Job drawing, mm, ordinate dimensions from the low corner. One solid piece. A direction names the side the tool comes from. Give positions to 0.01 mm unless a question says otherwise; leave off trailing zeros. Write each loop counter-clockwise with the first axis right and the second up, starting at its lowest first coordinate (ties: lowest second). Pieces come first, ordered by that corner, then holes. Notation, with made-up numbers: (6, 58) - (20, 58) arc R19 cw to (20, 82) - close; hole circle Ø11 at (-16, -10.75). An arc over 180 degrees is marked (long way). Use a Markdown table: item, result. Add a question column.
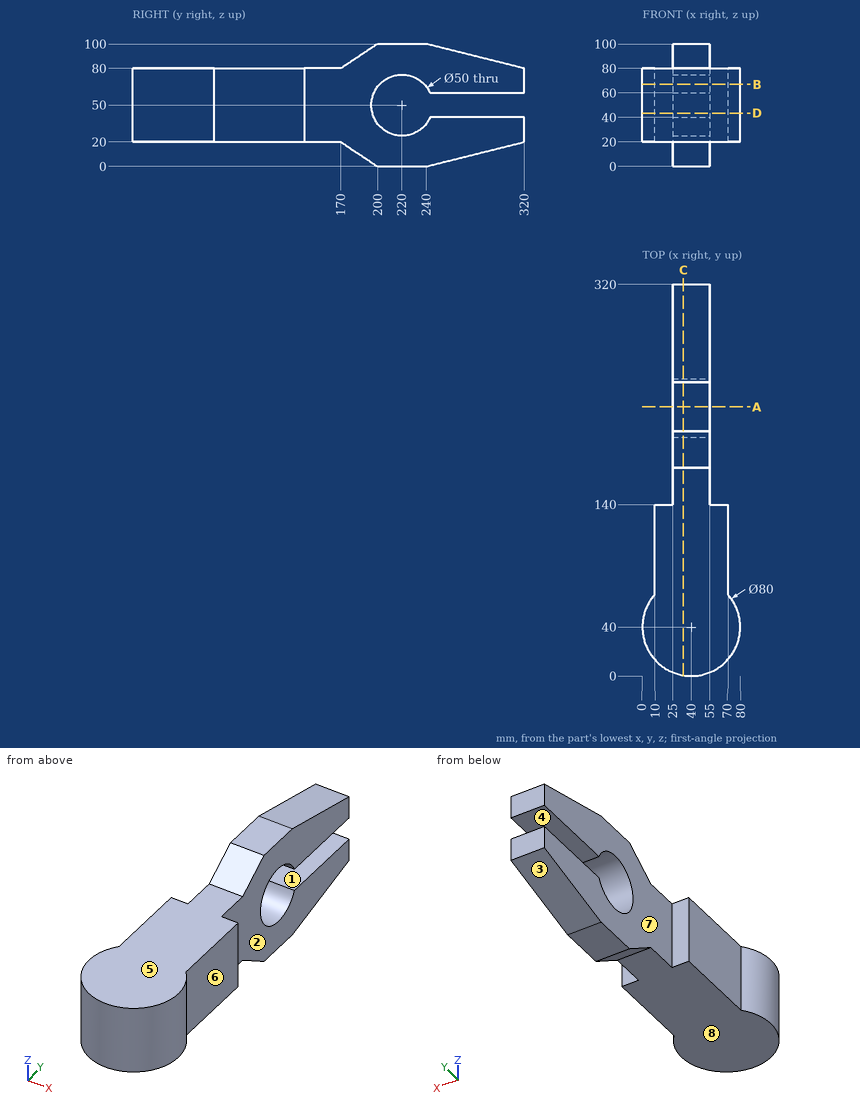
(1) Band-saw the part on A-A (y = 220). Write the cut outline in (x, z), then the cut area to 3 significant figures.
(2) Which spindle directions (+Z, -Z, +X, -X, +Y, -Y) get a long thin tool onto all of the face, cutting with end or side? Do the marked faces 4, 5, 6, 7 and 8. Say none if no direction does.
(3) Flat gauge pins, fed straight in: pin 1 (2 mm diameter, centred on y = 175, z = 23.5, fed in from -X); pin 2 (15 mm diameter, centred on x = 41, y = 293, fed in from -Z) (3 decimals); pin 3 (1.5 mm diameter, centred on x = 28.5, y = 162, fed in from +Z). Where does each tip first touch, or does it go through?
(4) Two-plate mould, pull along Z, no slides. Class the marked faces 1, 2 and 3: +Z half, -Z half, draft (parallel to the pull), parting line (faces both ways), or undercut.
(5) Probe probe 1 along Z at (x, y) = (44, 220); probe 2 along Z at (x, y) = (35.5, 165); probe 3 along X at (y, z) = (196, 62). List the from-to ranges inside material, lowest first. Write a range as [from, to].
(6) Band-saw the part on D-D (z = 43.5). Write the cut outline in (x, y), then the cut area to 3 significant figures.
(7) Band-saw the part on C-C (x = 33.5). Write the cut outline in (y, z).
(8) Band-saw the part on B-B (z = 67). Write the cut outline in (x, y).
Model answer:
| question | item | result |
|---|---|---|
| 1 | outline | (25, 0) - (55, 0) - (55, 25) - (25, 25) - close; (25, 75) - (55, 75) - (55, 100) - (25, 100) - close |
| 1 | area | 1,500 mm^2 |
| 2 | face 4 | +X, -X, +Y |
| 2 | face 5 | +Z, +X, -X, -Y |
| 2 | face 6 | +Z, -Z, +X, +Y |
| 2 | face 7 | +Z, -Z, -X, +Y |
| 2 | face 8 | -Z, +X, -X, -Y |
| 3 | pin 1 | stops at x = 25 |
| 3 | pin 2 | stops at z = 11.375 |
| 3 | pin 3 | stops at z = 80 |
| 4 | face 1 | undercut |
| 4 | face 2 | draft |
| 4 | face 3 | -Z half |
| 5 | probe 1 | z = [0, 25], [75, 100] |
| 5 | probe 2 | z = [20, 80] |
| 5 | probe 3 | x = [25, 55] |
| 6 | outline | (10, 66.46) arc R40 ccw (long way) to (70, 66.46) - (70, 140) - (55, 140) - (55, 195.86) - (25, 195.86) - (25, 140) - (10, 140) - close |
| 6 | area | 10,600 mm^2 |
| 7 | outline | (0.53, 20) - (170, 20) - (200, 0) - (240, 0) - (320, 20) - (320, 40) - (242.91, 40) arc R25 cw (long way) to (242.91, 60) - (320, 60) - (320, 80) - (240, 100) - (200, 100) - (170, 80) - (0.53, 80) - close |
| 8 | outline | (10, 66.46) arc R40 ccw (long way) to (70, 66.46) - (70, 140) - (55, 140) - (55, 201.67) - (25, 201.67) - (25, 140) - (10, 140) - close; (25, 238.33) - (55, 238.33) - (55, 320) - (25, 320) - close |
